For this review, take the finished solid that the model builds, in its own axes (mm). A direction names the side the tool comes from. Coordinates: 2 decimals unless noted, no trailing zeros. Put each result on its own line as item: value. Start each with the question number.
Item 1: Insertion check: P1, Ø21, axis at x = 0, z = 0, coming from the -Y side; P2, Ø4, axis at x = 0, z = -25, coming from the -Y side; P3, Ø7, axis at x = 0, z = 25, coming from the +Y side; P4, Ø4, axis at y = 12.5, z = -25.5, coming from the +X side. Each pin has a flat end and moves straight along its axis. Give the tip position at first contact, or say it passes through.
Item 2: Consider section A-A on x = 0. Give the number of separate pieces and of enclosed holes in the cut face, and give its area (3 significant figures).
Item 3: The part is to be moulded in two halves that separate along Z. For faces 5 (the flat face through (0, 21, 0)), 6 (the cylindrical face through (-21, 9, -28)), 7 (the cylindrical face through (-0.8, 11.32, -23.06)), say which applies: +Z half, -Z half, draft (parallel to the pull), parting line (faces both ways), or undercut.
Item 4: To check wall thickness, follow L1, parallel to Z at x = 0.5, y = 14.5; L2, parallel to Y at x = -5.5, z = 11.5; L3, parallel to X at y = 16.75, z = 11.5. State the ranges of each line that lie inside material, in increasing order.
Item 5: For faces 1 (the flat face through (9.3, 7.84, 9.3)), 2 (the flat face through (0, 17, 0)), 3 (the cylindrical face through (-0.8, 11.32, 26.94)), 4 (the cylindrical face through (-21.034, 18.782, -0.521)), list the 3-axis set-ups (+Z, -Z, +X, -X, +Y, -Y) from which the entire face can be reached by the end or side of a thin tool; tool diameter is ignored.
```python
from build123d import *

# Parameters (mm, degrees)
BOSS_EXTRUDE1_START       = 3
SKETCH1_R                 = 35
SKETCH1_R_2               = 14
BOSS_EXTRUDE1_DEPTH       = 18
BOSS_EXTRUDE2_START       = 18
SKETCH1_3_R               = 14
BOSS_EXTRUDE2_DEPTH       = 3
BOSS_EXTRUDE3_START       = 9
SKETCH1_4_R               = 14
SKETCH1_4_R_2             = 13
BOSS_EXTRUDE3_DEPTH       = 9
CUT_EXTRUDE1_REACH        = 54.669
SKETCH2_R                 = 2.1
SKETCH2_3_R               = 4
SKETCH2_3_R_2             = 2.1
CUT_EXTRUDE2_DEPTH        = 4.5
CHAMFER1_SIZE             = 0.5
BOSS_EXTRUDE4_START       = 3
BOSS_EXTRUDE4_OUTLINE_R   = 14
BOSS_EXTRUDE4_OUTLINE_R_2 = 13
BOSS_EXTRUDE4_DEPTH       = 4.84
BOSS_EXTRUDE5_START       = 1
SKETCH3_R                 = 13
BOSS_EXTRUDE5_DEPTH       = 1
SKETCH4_R                 = 35
CUT_EXTRUDE3_DEPTH        = 3.5
FILLET1_R                 = 10


# Read off the part's stored shape, not the designer's step: Boss-Extrude4
with BuildPart() as part:
    # Sketch1 → Boss-Extrude1 (new body)
    with BuildSketch(Plane(origin=(0, 0, 0), x_dir=(1, 0, 0), z_dir=(0, 1, 0)).offset(BOSS_EXTRUDE1_START)):
        with Locations(Location((0, 0, 0), (0, 0, 270))):
            Circle(SKETCH1_R)
        with Locations(Location((0, 0, 0), (0, 0, 270))):
            Circle(SKETCH1_R_2, mode=Mode.SUBTRACT)
    extrude(amount=BOSS_EXTRUDE1_DEPTH)

    # Sketch1<3> → Boss-Extrude2 (add)
    with BuildSketch(Plane(origin=(0, 0, 0), x_dir=(1, 0, 0), z_dir=(0, 1, 0)).offset(BOSS_EXTRUDE2_START)):
        with Locations(Location((0, 0, 0), (0, 0, 270))):
            Circle(SKETCH1_3_R)
    extrude(amount=BOSS_EXTRUDE2_DEPTH)

    # Sketch1<4> → Boss-Extrude3 (add)
    with BuildSketch(Plane(origin=(0, 0, 0), x_dir=(1, 0, 0), z_dir=(0, 1, 0)).offset(BOSS_EXTRUDE3_START)):
        with Locations(Location((0, 0, 0), (0, 0, 270))):
            Circle(SKETCH1_4_R)
        with Locations(Location((0, 0, 0), (0, 0, 270))):
            Circle(SKETCH1_4_R_2, mode=Mode.SUBTRACT)
    extrude(amount=BOSS_EXTRUDE3_DEPTH)

    # Sketch2 → Cut-Extrude1 (cut, up to next)
    with BuildSketch(Plane(origin=(0, 21, 0), x_dir=(1, 0, 0), z_dir=(0, 1, 0)), mode=Mode.PRIVATE) as cut_extrude1_sk1:
        with Locations(Location((0, -25, 0), (0, 0, 270))):
            Circle(SKETCH2_R)
    cut_extrude1_tool1 = extrude(cut_extrude1_sk1.sketch, amount=-CUT_EXTRUDE1_REACH, mode=Mode.PRIVATE) & part.part
    # Sketch2 → Cut-Extrude1 (cut, up to next)
    with BuildSketch(Plane(origin=(0, 21, 0), x_dir=(1, 0, 0), z_dir=(0, 1, 0)), mode=Mode.PRIVATE) as cut_extrude1_sk2:
        with Locations(Location((-25, 0, 0), (0, 0, 270))):
            Circle(SKETCH2_R)
    cut_extrude1_tool2 = extrude(cut_extrude1_sk2.sketch, amount=-CUT_EXTRUDE1_REACH, mode=Mode.PRIVATE) & part.part
    # Sketch2 → Cut-Extrude1 (cut, up to next)
    with BuildSketch(Plane(origin=(0, 21, 0), x_dir=(1, 0, 0), z_dir=(0, 1, 0)), mode=Mode.PRIVATE) as cut_extrude1_sk3:
        with Locations(Location((25, 0, 0), (0, 0, 270))):
            Circle(SKETCH2_R)
    cut_extrude1_tool3 = extrude(cut_extrude1_sk3.sketch, amount=-CUT_EXTRUDE1_REACH, mode=Mode.PRIVATE) & part.part
    # Sketch2 → Cut-Extrude1 (cut, up to next)
    with BuildSketch(Plane(origin=(0, 21, 0), x_dir=(1, 0, 0), z_dir=(0, 1, 0)), mode=Mode.PRIVATE) as cut_extrude1_sk4:
        with Locations(Location((0, 25, 0), (0, 0, 270))):
            Circle(SKETCH2_R)
    cut_extrude1_tool4 = extrude(cut_extrude1_sk4.sketch, amount=-CUT_EXTRUDE1_REACH, mode=Mode.PRIVATE) & part.part
    add(cut_extrude1_tool1.solids().sort_by_distance((0, 21, 25))[0], mode=Mode.SUBTRACT)
    add(cut_extrude1_tool2.solids().sort_by_distance((-25, 21, 0))[0], mode=Mode.SUBTRACT)
    add(cut_extrude1_tool3.solids().sort_by_distance((25, 21, 0))[0], mode=Mode.SUBTRACT)
    add(cut_extrude1_tool4.solids().sort_by_distance((0, 21, -25))[0], mode=Mode.SUBTRACT)

    # Sketch2<3> → Cut-Extrude2 (cut)
    # profile 1 of 4: a face of its own
    with BuildSketch(Plane(origin=(0, 21, 0), x_dir=(1, 0, 0), z_dir=(0, 1, 0))):
        with Locations(Location((0, -25, 0), (0, 0, 270))):
            Circle(SKETCH2_3_R)
        with Locations(Location((0, -25, 0), (0, 0, 270))):
            Circle(SKETCH2_3_R_2, mode=Mode.SUBTRACT)
    # profile 2 of 4: a face of its own
    with BuildSketch(Plane(origin=(0, 21, 0), x_dir=(1, 0, 0), z_dir=(0, 1, 0))):
        with Locations(Location((-25, 0, 0), (0, 0, 270))):
            Circle(SKETCH2_3_R)
        with Locations(Location((-25, 0, 0), (0, 0, 270))):
            Circle(SKETCH2_3_R_2, mode=Mode.SUBTRACT)
    # profile 3 of 4: a face of its own
    with BuildSketch(Plane(origin=(0, 21, 0), x_dir=(1, 0, 0), z_dir=(0, 1, 0))):
        with Locations(Location((0, 25, 0), (0, 0, 270))):
            Circle(SKETCH2_3_R)
        with Locations(Location((0, 25, 0), (0, 0, 270))):
            Circle(SKETCH2_3_R_2, mode=Mode.SUBTRACT)
    # profile 4 of 4: a face of its own
    with BuildSketch(Plane(origin=(0, 21, 0), x_dir=(1, 0, 0), z_dir=(0, 1, 0))):
        with Locations(Location((25, 0, 0), (0, 0, 270))):
            Circle(SKETCH2_3_R)
        with Locations(Location((25, 0, 0), (0, 0, 270))):
            Circle(SKETCH2_3_R_2, mode=Mode.SUBTRACT)
    extrude(amount=-CUT_EXTRUDE2_DEPTH, mode=Mode.SUBTRACT)

    # Chamfer1
    chamfer1_edges = [part.edges().sort_by_distance(p)[0] for p in [
        (0, 16.5, 22.9),
        (-25, 16.5, -2.1),
        (0, 16.5, -27.1),
        (25, 16.5, -2.1),
    ]]
    chamfer(chamfer1_edges, length=CHAMFER1_SIZE)

    # Boss-Extrude4 outline → Boss-Extrude4 (add)
    with BuildSketch(Plane(origin=(0, 0, 0), x_dir=(1, 0, 0), z_dir=(0, 1, 0)).offset(BOSS_EXTRUDE4_START)):
        Circle(BOSS_EXTRUDE4_OUTLINE_R)
        Circle(BOSS_EXTRUDE4_OUTLINE_R_2, mode=Mode.SUBTRACT)
    extrude(amount=BOSS_EXTRUDE4_DEPTH)

    # Sketch3 → Boss-Extrude5 (add)
    with BuildSketch(Plane.XZ.offset(-18).offset(BOSS_EXTRUDE5_START)):
        with Locations(Location((0, 0, 0), (0, 0, 270))):
            Circle(SKETCH3_R)
    extrude(amount=-BOSS_EXTRUDE5_DEPTH)

    # Sketch4 → Cut-Extrude3 (cut)
    with BuildSketch(Plane.XZ.offset(-3)):
        with Locations(Location((0, 0, 0), (0, 0, 270))):
            Circle(SKETCH4_R)
    extrude(amount=-CUT_EXTRUDE3_DEPTH, mode=Mode.SUBTRACT)

    # Fillet1
    # the kernel refuses this fillet: 10 mm, written as the material it takes off along each edge
    with BuildSketch(Plane(origin=(0, 21, 0), x_dir=(0, 0, 1), z_dir=(-1, 0, 0))) as fillet1_piece_1:
        with BuildLine():
            CenterArc((35 - FILLET1_R, -FILLET1_R), FILLET1_R, 0, 90)
            Line((35, -FILLET1_R), (35, 0))
            Line((35, 0), (35 - FILLET1_R, 0))
        make_face()
    revolve(axis=Axis((0, 21, 0), (0, 1, 0)), mode=Mode.SUBTRACT)


solid = part.part
```
Return value:
1. P1: y = 17
1. P2: through
1. P3: y = 16.5
1. P4: x = 25.82
2. separate pieces: 3
2. enclosed holes: 0
2. area: 542 mm^2
3. face 5: draft
3. face 6: parting line
3. face 7: undercut
4. L1: -34.36 to -27.04, -22.96 to -12.99, 12.99 to 22.96, 27.04 to 34.36
4. L2: 17 to 21
4. L3: -31.12 to -6.06, 6.06 to 31.12
5. face 1: none
5. face 2: -Y
5. face 3: +Y, -Y
5. face 4: +Y
